The listing builds one solid part. Answer for the finished solid, in the listing's coordinates (mm). A direction names the side the tool comes from. Coordinates: 2 decimals unless noted, no trailing zeros. Write each loop counter-clockwise with the first axis right and the second up, starting at its lowest first coordinate (ties: lowest second). Pieces come first, ordered by that corner, then holes.
from build123d import *

# Parameters (mm, degrees)
BOSS_EXTRUDE1_DEPTH = 10
SKETCH2_W           = 2
SKETCH2_H           = 0.5
CUT_EXTRUDE1_DEPTH  = 10
CUT_EXTRUDE2_DEPTH  = 0.5
FILLET1_R           = 1.5
FILLET2_R           = 1.5
BOSS_EXTRUDE2_DEPTH = 1


with BuildPart() as part:
    # Sketch1 → Boss-Extrude1 (new body)
    with BuildSketch(Plane(origin=(0, 0, 0), x_dir=(1, 0, 0), z_dir=(0, 1, 0))):
        with BuildLine():
            Line((-8, 7.5), (8, 7.5))
            ThreePointArc((8, 7.5), (9.414213562, 6.914213562), (10, 5.5))
            Line((10, 5.5), (10, -5.5))
            ThreePointArc((10, -5.5), (9.414213562, -6.914213562), (8, -7.5))
            Line((8, -7.5), (-8, -7.5))
            ThreePointArc((-8, -7.5), (-9.414213562, -6.914213562), (-10, -5.5))
            Line((-10, -5.5), (-10, 5.5))
            ThreePointArc((-10, 5.5), (-9.414213562, 6.914213562), (-8, 7.5))
        make_face()
    extrude(amount=BOSS_EXTRUDE1_DEPTH)

    # Sketch2 → Cut-Extrude1 (cut)
    with BuildSketch(Plane(origin=(0, 10, 0), x_dir=(1, 0, 0), z_dir=(0, 1, 0))):
        with Locations((-5, 7.25)):
            Rectangle(SKETCH2_W, SKETCH2_H)
        with Locations((5, 7.25)):
            Rectangle(SKETCH2_W, SKETCH2_H)
        with Locations((5, -7.25)):
            Rectangle(SKETCH2_W, SKETCH2_H)
        with Locations((-5, -7.25)):
            Rectangle(SKETCH2_W, SKETCH2_H)
    extrude(amount=-CUT_EXTRUDE1_DEPTH, mode=Mode.SUBTRACT)

    # Sketch3 → Cut-Extrude2 (cut)
    with BuildSketch(Plane(origin=(0, 10, 0), x_dir=(1, 0, 0), z_dir=(0, 1, 0))):
        Polygon((-6, 7), (-6, 5.986822399), (-4.02260562, 5.986822399), (-4, 6), (-4, 7), align=None)
        Polygon((4, 7), (4, 6), (4.02260562, 5.986822399), (6, 5.986822399), (6, 7), align=None)
        Polygon((6, -7), (4, -7), (4, -6), (4.02260562, -5.986822399), (6, -5.986822399), align=None)
        Polygon((-4, -7), (-4, -6), (-4.02260562, -5.986822399), (-6, -5.986822399), (-6, -7), align=None)
    extrude(amount=-CUT_EXTRUDE2_DEPTH, mode=Mode.SUBTRACT)

    # Fillet1
    fillet1_edges = [part.edges().sort_by_distance(p)[0] for p in [
        (-9.414213562, 10, 6.914213562),
        (-10, 10, 0),
        (-9.414213562, 10, -6.914213562),
        (7, 10, -7.5),
        (-7, 10, -7.5),
        (9.414213562, 10, -6.914213562),
        (10, 10, 0),
        (9.414213562, 10, 6.914213562),
        (7, 10, 7.5),
        (-7, 10, 7.5),
        (0, 10, 7.5),
        (0, 10, -7.5),
    ]]
    fillet(fillet1_edges, radius=FILLET1_R)

    # Fillet2
    # the kernel refuses this fillet: 1.5 mm, written as the material it takes off along each edge
    with BuildSketch(Plane(origin=(2.25, 0, -7.5), x_dir=(0, 0, 1), z_dir=(1, 0, 0)), Plane(origin=(8, 0, 7.5), x_dir=(0, 0, -1), z_dir=(-1, 0, 0)), Plane(origin=(-2.25, 0, 7.5), x_dir=(0, 0, -1), z_dir=(-1, 0, 0))) as fillet2_piece_1:
        with BuildLine():
            CenterArc((FILLET2_R, -FILLET2_R), FILLET2_R, 90, 90)
            Line((0, -FILLET2_R), (0, 0))
            Line((0, 0), (FILLET2_R, 0))
        make_face()
    extrude(amount=5.75, mode=Mode.SUBTRACT)
    with BuildSketch(Plane(origin=(8, 0, -5.5), x_dir=(0, 0, -1), z_dir=(-1, 0, 0))) as fillet2_piece_2:
        with BuildLine():
            CenterArc((2 - FILLET2_R, -FILLET2_R), FILLET2_R, 0, 90)
            Line((2, -FILLET2_R), (2, 0))
            Line((2, 0), (2 - FILLET2_R, 0))
        make_face()
    revolve(axis=Axis((8, 0, -5.5), (0, -1, 0)), revolution_arc=90, mode=Mode.SUBTRACT)
    with BuildSketch(Plane(origin=(10, 0, -5.5), x_dir=(-1, 0, 0), z_dir=(0, 0, 1)), Plane(origin=(-10, 0, 5.5), x_dir=(1, 0, 0), z_dir=(0, 0, -1))) as fillet2_piece_3:
        with BuildLine():
            CenterArc((FILLET2_R, -FILLET2_R), FILLET2_R, 90, 90)
            Line((0, -FILLET2_R), (0, 0))
            Line((0, 0), (FILLET2_R, 0))
        make_face()
    extrude(amount=11, mode=Mode.SUBTRACT)
    with BuildSketch(Plane(origin=(8, 0, 5.5), x_dir=(1, 0, 0), z_dir=(0, 0, -1))) as fillet2_piece_4:
        with BuildLine():
            CenterArc((2 - FILLET2_R, -FILLET2_R), FILLET2_R, 0, 90)
            Line((2, -FILLET2_R), (2, 0))
            Line((2, 0), (2 - FILLET2_R, 0))
        make_face()
    revolve(axis=Axis((8, 0, 5.5), (0, -1, 0)), revolution_arc=90, mode=Mode.SUBTRACT)
    with BuildSketch(Plane(origin=(7.75, 0, 7.5), x_dir=(0, 0, -1), z_dir=(-1, 0, 0)), Plane(origin=(-7.75, 0, -7.5), x_dir=(0, 0, 1), z_dir=(1, 0, 0))) as fillet2_piece_5:
        with BuildLine():
            CenterArc((FILLET2_R, -FILLET2_R), FILLET2_R, 90, 90)
            Line((0, -FILLET2_R), (0, 0))
            Line((0, 0), (FILLET2_R, 0))
        make_face()
    extrude(amount=15.5, mode=Mode.SUBTRACT)
    with BuildSketch(Plane(origin=(-8, 0, -7.5), x_dir=(0, 1, 0), z_dir=(1, 0, 0))) as fillet2_piece_6:
        with BuildLine():
            CenterArc((FILLET2_R, FILLET2_R), FILLET2_R, 180, 90)
            Line((0, FILLET2_R), (0, 0))
            Line((0, 0), (FILLET2_R, 0))
        make_face()
    extrude(amount=5.75, mode=Mode.SUBTRACT)
    with BuildSketch(Plane(origin=(-8, 0, 5.5), x_dir=(0, 0, 1), z_dir=(1, 0, 0))) as fillet2_piece_7:
        with BuildLine():
            CenterArc((2 - FILLET2_R, -FILLET2_R), FILLET2_R, 0, 90)
            Line((2, -FILLET2_R), (2, 0))
            Line((2, 0), (2 - FILLET2_R, 0))
        make_face()
    revolve(axis=Axis((-8, 0, 5.5), (0, -1, 0)), revolution_arc=90, mode=Mode.SUBTRACT)
    with BuildSketch(Plane(origin=(-8, 0, -5.5), x_dir=(-1, 0, 0), z_dir=(0, 0, 1))) as fillet2_piece_8:
        with BuildLine():
            CenterArc((2 - FILLET2_R, -FILLET2_R), FILLET2_R, 0, 90)
            Line((2, -FILLET2_R), (2, 0))
            Line((2, 0), (2 - FILLET2_R, 0))
        make_face()
    revolve(axis=Axis((-8, 0, -5.5), (0, -1, 0)), revolution_arc=90, mode=Mode.SUBTRACT)

    # Sketch4 → Boss-Extrude2 (add)
    with BuildSketch(Plane(origin=(0, 10, 0), x_dir=(1, 0, 0), z_dir=(0, 1, 0))):
        Polygon((-1, 4), (1, 4), (1, 1), (4, 1), (4, -1), (1, -1), (1, -4), (-1, -4), (-1, -1), (-4, -1), (-4, 1), (-1, 1), align=None)
    extrude(amount=BOSS_EXTRUDE2_DEPTH)


solid = part.part
Q1. The part is cut by section C-C, the plane x = 5. Write down the section's boundary in (y, z), then the cut area to 3 significant figures.
Answers below:
outline: (0, -6) arc R1.5 ccw to (0.38, -7) - (9.5, -7) - (9.5, -5.99) - (10, -5.99) - (10, 5.99) - (9.5, 5.99) - (9.5, 7) - (0.38, 7) arc R1.5 ccw to (0, 6) - close
area: 139 mm2
Q2. Which of the six approach directions +Z, -Z, +X, -X, +Y, -Y give full straight-line access (tool end or side, diameter ignored) to faces 4 (the face through (-6, 6.3, -7.2)), 5 (the face through (-2.5, 10.5, -1)), 6 (the face through (5, 5, 7))?
Answers below:
face 4: -Z, +Y
face 5: -Z, -X, +Y
face 6: +Z, +Y, -Y
Q3. The part is cut by section D-D, the plane z = -0.5. Write down the section's boundary in (x, y), then the cut area to 3 significant figures.
Answers below:
outline: (-10, 1.5) arc R1.5 ccw to (-8.5, 0) - (8.5, 0) arc R1.5 ccw to (10, 1.5) - (10, 8.5) arc R1.5 ccw to (8.5, 10) - (4, 10) - (4, 11) - (-4, 11) - (-4, 10) - (-8.5, 10) arc R1.5 ccw to (-10, 8.5) - close
area: 206 mm2
Q4. Find the intervals of material crossed by probe 1 along Z at (x, y) = (-5, 6.75); probe 2 along Y at (x, z) = (7.5, -2); probe 3 along Z at (x, y) = (5, 9.75), in increasing order.
Answers below:
probe 1: z = -7 to 7
probe 2: y = 0 to 10
probe 3: z = -5.99 to 5.99
Q5. The part is cut by section B-B, the plane y = 2.25. Write down the section's boundary in (x, z), then the cut area to 3 significant figures.
Answers below:
outline: (-10, -5.5) arc R2 ccw to (-8, -7.5) - (-6, -7.5) - (-6, -7) - (-4, -7) - (-4, -7.5) - (4, -7.5) - (4, -7) - (6, -7) - (6, -7.5) - (8, -7.5) arc R2 ccw to (10, -5.5) - (10, 5.5) arc R2 ccw to (8, 7.5) - (6, 7.5) - (6, 7) - (4, 7) - (4, 7.5) - (-4, 7.5) - (-4, 7) - (-6, 7) - (-6, 7.5) - (-8, 7.5) arc R2 ccw to (-10, 5.5) - close
area: 293 mm2
Q6. Given pin 1 (0.8 mm diameter, centred on x = 4.5, z = 6.5, fed in from +Y); pin 2 (1.7 mm diameter, centred on y = 6.5, z = -6.5, fed in from -X); pin 3 (1.7 mm diameter, centred on y = 6, z = -6.5, fed in from +X), each flat-ended and moving along its own axis, determine where each tip first touches the part or whether it passes through.
Answers below:
pin 1: stops at y = 9.5
pin 2: stops at x = -9.99
pin 3: stops at x = 9.99
Q7. The part is cut by section A-A, the plane z = -2.25. Write down the section's boundary in (x, y).
Answers below:
outline: (-10, 1.5) arc R1.5 ccw to (-8.5, 0) - (8.5, 0) arc R1.5 ccw to (10, 1.5) - (10, 8.5) arc R1.5 ccw to (8.5, 10) - (1, 10) - (1, 11) - (-1, 11) - (-1, 10) - (-8.5, 10) arc R1.5 ccw to (-10, 8.5) - close
Q8. Determine the mould class of faces 1 (the face through (4, 6.3, -7.2)), 2 (the face through (7, 5, -7.5)), 3 (the face through (-10, 5, 0)) for opening direction X: released by +X, released by -X, zero draft, split by the parting line, or undercut.
Answers below:
face 1: undercut
face 2: zero draft
face 3: released by -X
